Autodesk Inventor part; units mm, degrees
ref_plane "YZ Plane" through (0, 0, 0) normal (1, 0, 0) x (0, 1, 0)
ref_plane "XZ Plane" through (0, 0, 0) normal (0, 1, 0) x (-1, 0, 0)
ref_plane "XY Plane" through (0, 0, 0) normal (0, 0, 1) x (1, 0, 0)
sketch "Sketch1" plane through (0, 0, 0) normal (0, 1, 0) x (-1, 0, 0)
  line L0 (0, 0) -> (0, -26)
  line L1 (0, -26) -> (1.5, -25.8688)
  line L2 (-5, -13) -> (15, -13) construction
  line L3 (0, 0) -> (1.5, -0.1312)
  arc A0 (1.5, -25.8688) -> (5.6905, -21.6131) centre (1.0988, -21.2827) ccw
  arc A1 (5.6905, -4.3869) -> (1.5, -0.1312) centre (1.0988, -4.7173) ccw
  arc A2 (5.6905, -21.6131) -> (6, -13) centre (-114, -13) ccw
  arc A3 (6, -13) -> (5.6905, -4.3869) centre (-114, -13) ccw
  dimension "d0" = 26
  dimension "d1" = 85
  dimension "d2" = 1.5
  dimension "d3" = 6
  dimension "d4" = 120
extrude "Extrusion1" add sketch "Sketch1" along normal blind 9.5
sketch "Sketch2" plane through (0, 0, 0) normal (1, 0, 0) x (0, 0, -1)
  circle A0 centre (7, 6) radius 2
  circle A1 centre (19, 6) radius 2
  line L0 (0, 0) -> (26, 0) construction
  line L1 (26, 0) -> (26, 9.5) construction
  line L2 (0, 9.5) -> (1, 9.5) construction
  line L3 (0, 0) -> (0, 9.5) construction
  line L4 (1, 9.5) -> (1, 1)
  line L5 (1, 1) -> (25, 1)
  line L6 (25, 1) -> (25, 9.5)
  line L7 (0, 0) -> (0, 9.5) construction
  line L8 (0, 9.5) -> (1, 9.5) construction
  line L9 (26, 0) -> (26, 9.5) construction
  line L10 (1, 9.5) -> (25, 9.5)
  line L11 (25, 9.5) -> (26, 9.5) construction
  dimension "d7" = 1
  dimension "d8" = 1
  dimension "d9" = 1
extrude "Extrusion2" cut sketch "Sketch2" against normal blind 0.2
sketch "Sketch3" plane through (0, 6, -7) normal (1, 0, 0) x (0, 0, -1)
  circle A0 centre (0, 0) radius 2
  circle A1 centre (0, 0) radius 2
  circle A2 centre (12, 0) radius 2
  point P0 (-7, -6)
extrude "Extrusion3" add sketch "Sketch3" along normal blind 2.5
sketch "Sketch4" plane through (2.5, 6, -7) normal (1, 0, 0) x (0, 0, -1)
  circle A0 centre (12, 0) radius 2
  point P0 (-7, -6)
  point P1 (0, 0)
hole "Hole1" at (2.5, 6, -7) at (2.5, 6, -19) direction (-1, 0, 0) diameter 1.221 depth 5.3 tip angle 118
sketch "Sketch5" plane through (0, 0, 0) normal (1, 0, 0) x (0, 0, -1)
  line L0 (21.6131, 9.5) -> (4.3869, 9.5) construction
  line L1 (13, 9.5) -> (13, -3) construction
  line L2 (10.5, 8) -> (13, 8) construction
  arc A0 (15.5, 3.101) -> (15.5, 8) centre (13, 5.5505) ccw
  line L3 (21.6131, 0) -> (4.3869, 0) construction
  line L4 (10.5, 0) -> (10.5, 3.101) construction
  line L5 (15.5, 0) -> (15.5, 3.101)
  line L6 (13, 9.0505) -> (13, 8) construction
  arc A1 (13, 2.0505) -> (15.5, 3.101) centre (13, 5.5505) ccw construction
  arc A2 (13, 9.0505) -> (13, 2.0505) centre (13, 5.5505) ccw construction
  arc A3 (15.5, 8) -> (13, 9.0505) centre (13, 5.5505) ccw construction
  line L7 (13, 8) -> (15.5, 8)
  line L8 (13, 8) -> (13, 0)
  line L9 (13, 0) -> (15.5, 0)
  point P0 (0, 0)
  dimension "d24" = 1.5
  dimension "d25" = 5
  dimension "d26" = 7
  dimension "d27" = 5
revolve "Revolution1" cut sketch "Sketch5" angle 360 about axis through (0, 8, -13) along (0, -1, 0)
equation "\"d9\" = d7"
The listing builds one solid part. Answer for the finished solid, in the listing's coordinates (mm). A direction names the side the tool comes from. Round coordinates to 2 decimals unless told otherwise and drop trailing zeros. Write each loop counter-clockwise with the first axis right and the second up, starting at its lowest first coordinate (ties: lowest second). Pieces come first, ordered by that corner, then holes. Notation, with made-up numbers: (62.25, 85.25) -> (96.25, 85.25) arc R10 cw to (96.25, 99.25) -> close; hole circle Ø11 at (-33.5, 13.5). An arc over 180 degrees is marked (long way). Answer as a JSON object with one key per item and string values. Group by question number.
Q1. Straight lines are drawn through the part: line 1 along Z through (x, y) = (0.25, 5.75); line 2 along Z through (x, y) = (1, 5.5); line 3 along Y through (x, z) = (0.55, -7). For each, find the intervals that lie inside material, in ascending order.
Q2. Section D-D (y = 2) is taken. Write down the section's boundary in (x, z), plus the area to 3 significant figures.
Q3. Section A-A (y = 8.75) is taken. Write down the section's boundary in (x, z).
Q4. Each of these flat-tipped pins is pushed along its axis until it touches: pin 1 Ø1.5 at (x, y) = (-4.5, 7) entering from +Z; pin 2 Ø2 at (y, z) = (3.5, -16.5) entering from +X; pin 3 Ø0.7 at (x, z) = (-1.5, -13) entering from -Y. Where does it stop, or does it pass through?
Q5. Determine the mould class of faces 1 (the face through (-3.1, 5.96, -19.1)), 2 (the face through (2.5, 6, -20)), 3 (the face through (-0.2, 3, -10)), 4 (the face through (-3, 9.5, -13)) for opening direction Y: pulls with the +Y half, pulls with the -Y half, needs draft (parallel to the pull), parting line crosses it, or undercut.
Q6. Section C-C (z = -14.25) is taken. Write down the section's boundary in (x, y), plus the area to 3 significant figures.
Q7. Which of the six approach directions +Z, -Z, +X, -X, +Y, -Y give full straight-line access (tool end or side, diameter ignored) to faces 5 (the face through (-4.35, 4.68, -1.46)), 6 (the face through (-2.5, 1.6, -13.1)), 7 (the face through (-0.187, 5.485, -7.328)), 8 (the face through (0, 0.5, -23.1))?
Q8. Section B-B (x = -0.5) is taken. Write down the section's boundary in (y, z).
Check values:
{
 "1": {"line 1": "-20.98 to -19.56, -18.44 to -17.02, -8.98 to -7.56, -6.44 to -5.02", "line 2": "-20.94 to -19.35, -18.65 to -17.06, -8.94 to -7.35, -6.65 to -5.06", "line 3": "4 to 5.39, 6.61 to 8"},
 "2": {"outline": "(-6, -13) arc R120 ccw to (-5.69, -21.61) arc R4.6 ccw to (-1.5, -25.87) -> (0, -26) -> (0, -25) -> (-0.2, -25) -> (-0.2, -15.49) arc R2.5 cw to (-0.2, -10.51) -> (-0.2, -1) -> (0, -1) -> (0, 0) -> (-1.5, -0.13) arc R4.6 ccw to (-5.69, -4.39) arc R120 ccw to start", "area": "128 mm^2"},
 "3": {"outline": "(-6, -13) arc R120 ccw to (-5.69, -21.61) arc R4.6 ccw to (-1.5, -25.87) -> (0, -26) -> (0, -25) -> (-0.2, -25) -> (-0.2, -1) -> (0, -1) -> (0, 0) -> (-1.5, -0.13) arc R4.6 ccw to (-5.69, -4.39) arc R120 ccw to start"},
 "4": {"pin 1": "z = -0.95", "pin 2": "x = -0.2", "pin 3": "y = 8"},
 "5": {"face 1": "undercut", "face 2": "needs draft", "face 3": "undercut", "face 4": "pulls with the +Y half"},
 "6": {"outline": "(-5.99, 0) -> (-2.17, 0) -> (-2.17, 3.1) arc R3.27 cw to (-2.17, 8) -> (-0.2, 8) -> (-0.2, 9.5) -> (-5.99, 9.5) -> close", "area": "35.6 mm^2"},
 "7": {"face 5": "+Z, -X, +Y, -Y", "face 6": "+X, -Y", "face 7": "+X", "face 8": "-Z, +X, -Y"},
 "8": {"outline": "(0, -25.96) -> (9.5, -25.96) -> (9.5, -0.04) -> (0, -0.04) -> (0, -10.55) -> (3.1, -10.55) arc R3.46 cw to (8, -10.55) -> (8, -15.45) arc R3.46 cw to (3.1, -15.45) -> (0, -15.45) -> close; hole circle Ø1.22 at (6, -19); hole circle Ø1.22 at (6, -7)"}
}
